from build123d import *

# Parameters (mm, degrees)
SKETCH1_W                 = 59
SKETCH1_H                 = 79
EXTRUDE1_DEPTH            = 1.778
F_2_CLEARANCE_HOLE1_D     = 2.4384
F_2_CLEARANCE_HOLE1_DEPTH = 6.35
F_2_CLEARANCE_HOLE1_TIP   = 0.732569267


with BuildPart() as part:
    # Sketch1 → Extrude1 (new body)
    with BuildSketch(Plane.XY):
        with Locations((0, 1)):
            Rectangle(SKETCH1_W, SKETCH1_H)
    extrude(amount=EXTRUDE1_DEPTH)

    # #2 Clearance Hole1
    with Locations(Plane(origin=(-25.055, -28.34, 1.778), x_dir=(1, 0, 0), z_dir=(0, 0, 1))):
        with Locations((0, 0), (-0.254, 35.179), (49.784, 37.084), (51.308, -6.985)):
            Hole(F_2_CLEARANCE_HOLE1_D / 2, depth=F_2_CLEARANCE_HOLE1_DEPTH)
            with Locations((0, 0, -(F_2_CLEARANCE_HOLE1_DEPTH + F_2_CLEARANCE_HOLE1_TIP / 2))):  # 118° drill point
                Cone(0, F_2_CLEARANCE_HOLE1_D / 2, F_2_CLEARANCE_HOLE1_TIP, mode=Mode.SUBTRACT)


solid = part.part
Read the model definition and answer for the solid it produces. Units are mm, in the model's axes. Round coordinates to 2 decimals unless told otherwise and drop trailing zeros. Write each loop counter-clockwise with the first axis right and the second up, starting at its lowest first coordinate (ties: lowest second). Pieces come first, ordered by that corner, then holes. Notation, with made-up numbers: (55.25, 27) - (63.25, 27) arc R28 ccw to (63.25, 58) - close; hole circle Ø8 at (60, -34). An arc over 180 degrees is marked (long way). Use a Markdown table: item, result.
(1) The mould has two halves that part along Y. Classify faces 1 (the flat face through (0, -38.5, 1)), 2 (the flat face through (-29.5, 0, 1)), 3 (the cylindrical face through (27.22, -36.07, 0.88)), 4 (the cylindrical face through (-25.04, 5.65, 0.88)): released by +Y, released by -Y, zero draft, split by the parting line, or undercut.
Reported:
| item | result |
|---|---|
| face 1 | released by -Y |
| face 2 | zero draft |
| face 3 | undercut |
| face 4 | undercut |
(2) A straight line is drawn through the part: line 1 along Y through (x, z) = (-24.5, 0.8). Find the intervals that lie inside material, in ascending order. Write a range as [from, to].
Reported:
| item | result |
|---|---|
| line 1 | [-38.5, -29.43], [-27.25, 5.93], [7.75, 40.5] |
(3) The part is cut by section A-A (y = -28.34). Write down the section's boundary in (x, z), then the cut area to 3 significant figures.
Reported:
| item | result |
|---|---|
| outline | (-29.5, 0) - (-26.27, 0) - (-26.27, 1.78) - (-29.5, 1.78) - close; (-23.84, 0) - (29.5, 0) - (29.5, 1.78) - (-23.84, 1.78) - close |
| area | 101 mm2 |
